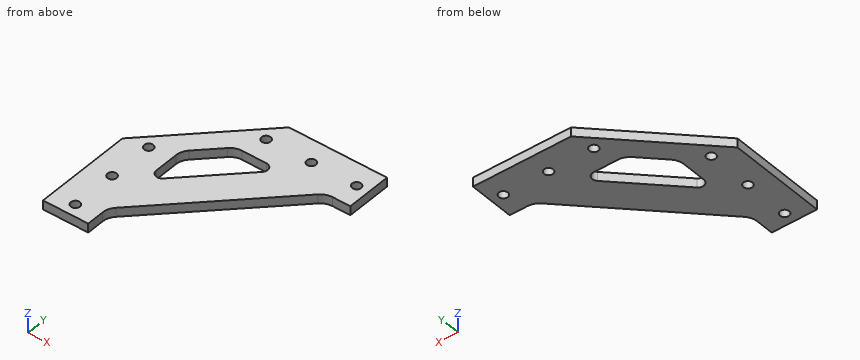
from build123d import *

# Parameters (mm, degrees)
EXTRUDE_1_DEPTH     = 3
SKETCH_2_R          = 1.5
CUT_EXTRUDE_1_DEPTH = 10


with BuildPart() as part:
    # 草图1 → 凸台-拉伸1 (new body)
    with BuildSketch(Plane.XY):
        with BuildLine():
            Line((32.5, 0), (32.5, -15))
            Line((32.5, -15), (26.571067812, -15))
            ThreePointArc((26.571067812, -15), (24.65765065, -15.380602337), (23.035533906, -16.464466094))
            Line((23.035533906, -16.464466094), (-14.035533906, -53.535533906))
            ThreePointArc((-14.035533906, -53.535533906), (-15.119397663, -55.15765065), (-15.5, -57.071067812))
            Line((-15.5, -57.071067812), (-15.5, -63))
            Line((-15.5, -63), (-30.5, -63))
            Line((-30.5, -63), (-30.5, -30.5))
            Line((-30.5, -30.5), (0, 0))
            Line((0, 0), (32.5, 0))
        make_face()
        with BuildLine():
            Line((-12.085786438, -36.585786438), (6.085786438, -18.414213562))
            ThreePointArc((6.085786438, -18.414213562), (6.51933194, -16.234633135), (4.671572875, -15))
            Line((4.671572875, -15), (-3.428932188, -15))
            ThreePointArc((-3.428932188, -15), (-5.34234935, -15.380602337), (-6.964466094, -16.464466094))
            Line((-6.964466094, -16.464466094), (-14.035533906, -23.535533906))
            ThreePointArc((-14.035533906, -23.535533906), (-15.119397663, -25.15765065), (-15.5, -27.071067812))
            Line((-15.5, -27.071067812), (-15.5, -35.171572875))
            ThreePointArc((-15.5, -35.171572875), (-14.265366865, -37.01933194), (-12.085786438, -36.585786438))
        make_face(mode=Mode.SUBTRACT)
    extrude(amount=EXTRUDE_1_DEPTH)

    # 草图2 → 切除-拉伸1 (cut)
    with BuildSketch(Plane.XY.offset(3)):
        with Locations((28.5, -7.5)):
            Circle(SKETCH_2_R)
        with Locations((13.5, -7.5)):
            Circle(SKETCH_2_R)
        with Locations((-1.5, -7.5)):
            Circle(SKETCH_2_R)
        with Locations((-23, -29)):
            Circle(SKETCH_2_R)
        with Locations((-23, -44)):
            Circle(SKETCH_2_R)
        with Locations((-23, -59)):
            Circle(SKETCH_2_R)
    extrude(amount=-CUT_EXTRUDE_1_DEPTH, mode=Mode.SUBTRACT)


solid = part.part
Geometry check sheet. Reference: the model listing, model coordinates, mm. Give positions to 0.01 mm unless a question says otherwise; leave off trailing zeros. Write each loop counter-clockwise with the first axis right and the second up, starting at its lowest first coordinate (ties: lowest second). Pieces come first, ordered by that corner, then holes.
1) Cross-section at C-C (x = 28.5). Record the boundary of the cut face in (y, z), plus the area to 3 significant figures.
Values follow:
outline: (-15, 0) - (-9, 0) - (-9, 3) - (-15, 3) - close; (-6, 0) - (0, 0) - (0, 3) - (-6, 3) - close
area: 36.0 mm2
2) Cross-section at A-A (y = -44). Record the boundary of the cut face in (x, z).
Values follow:
outline: (-30.5, 0) - (-24.5, 0) - (-24.5, 3) - (-30.5, 3) - close; (-21.5, 0) - (-4.5, 0) - (-4.5, 3) - (-21.5, 3) - close
3) Cross-section at B-B (x = -1.5). Record the boundary of the cut face in (y, z), plus the area to 3 significant figures.
Values follow:
outline: (-41, 0) - (-26, 0) - (-26, 3) - (-41, 3) - close; (-15, 0) - (-9, 0) - (-9, 3) - (-15, 3) - close; (-6, 0) - (-1.5, 0) - (-1.5, 3) - (-6, 3) - close
area: 76.5 mm2
4) Cross-section at D-D (z = 1.85). Record the boundary of the cut face in (x, y).
Values follow:
outline: (-30.5, -63) - (-15.5, -63) - (-15.5, -57.07) arc R5 cw to (-14.04, -53.54) - (23.04, -16.46) arc R5 cw to (26.57, -15) - (32.5, -15) - (32.5, 0) - (0, 0) - (-30.5, -30.5) - close; hole circle Ø3 at (-23, -59); hole circle Ø3 at (-23, -44); hole circle Ø3 at (-23, -29); hole (-15.5, -35.17) arc R2 ccw to (-12.09, -36.59) - (6.09, -18.41) arc R2 ccw to (4.67, -15) - (-3.43, -15) arc R5 ccw to (-6.96, -16.46) - (-14.04, -23.54) arc R5 ccw to (-15.5, -27.07) - close; hole circle Ø3 at (-1.5, -7.5); hole circle Ø3 at (13.5, -7.5); hole circle Ø3 at (28.5, -7.5)
5) Thickness scan on line 1 (Y direction, x = -23, z = 2.2); line 2 (Y direction, x = -24, z = 2.8); line 3 (Y direction, x = -15, z = 2.6). Record the ranges inside material, lowest first.
Values follow:
line 1: y = -63 to -60.5, -57.5 to -45.5, -42.5 to -30.5, -27.5 to -23
line 2: y = -63 to -60.12, -57.88 to -45.12, -42.88 to -30.12, -27.88 to -24
line 3: y = -54.89 to -36.49, -24.89 to -15
6) Go/stop test with flat-tipped pins: pin 1 Ø1 at (x, y) = (14.5, -7) entering from -Z; pin 2 Ø1.5 at (y, z) = (-33, 2) entering from +X; pin 3 Ø0.9 at (x, z) = (30, 1) entering from -Y; pin 4 Ø1.5 at (x, z) = (-0.5, 2) entering from -Y. Record where each tip stops, or that it passes through.
Values follow:
pin 1: stops at z = 0
pin 2: stops at x = 7.25
pin 3: stops at y = -15
pin 4: stops at y = -40.75
